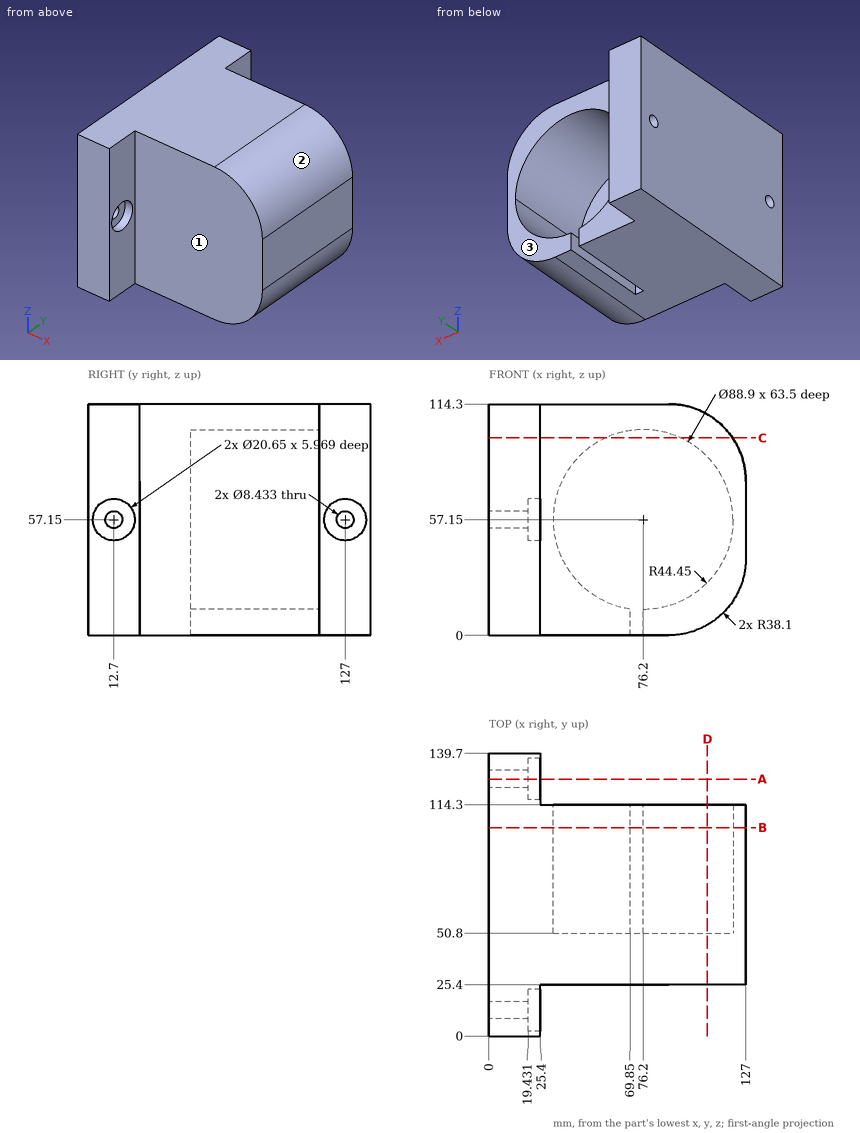
Check sheet for the drawn part. Datum: minimum x, y, z corner. Units: mm. A direction names the side the tool comes from. Give positions to 0.01 mm unless a question says otherwise; leave off trailing zeros. Order: outer loops, then holes, each group sorted by start corner. A loop starts at its lowest first (then second) coordinate and runs counter-clockwise, first axis right, second up. Notation, with made-up numbers: (-33, -18) - (4, -18) arc R15 ccw to (4, -13) - close; hole circle Ø9 at (-13.5, 19). An arc over 180 degrees is marked (long way). Answer in a Markdown table with one row per item. Add a question column.
Q1. Cross-section at B-B, the plane y = 103. Enter the section's corners in (x, z).
Q2. Gauge pin test, flat ends, axial feed: pin 1 (12 mm diameter, centred on y = 16, z = 58.5, fed in from +X); pin 2 (20.5 mm diameter, centred on y = 15, z = 57, fed in from +X); pin 3 (4 mm diameter, centred on x = 85, z = 21, fed in from -Y); pin 4 (4 mm diameter, centred on y = 73, z = 9, fed in from -X). Record the tip position at first contact, or that the pin passes through.
Q3. Tool access check on the marked faces 1, 2 and 3. Record the directions out of +Z, -Z, +X, -X, +Y, -Y that give a thin tool (end or side, any length) a straight path to the whole face; none if there is none.
Q4. Cross-section at D-D, the plane x = 108. Enter the section's corners in (y, z).
Q5. Cross-section at A-A, the plane y = 127. Enter the section's corners in (x, z) (1 decimal).
Q6. Material ranges on probe 1 along Y at (x, z) = (24, 57); probe 2 along X at (y, z) = (101.5, 82.5) (1 decimal); probe 3 along X at (y, z) = (93, 57), recorded low to high. Write a range as from..to.
Q7. Cross-section at C-C, the plane z = 97.5. Enter the section's corners in (x, y).
Check values:
| question | item | result |
|---|---|---|
| 1 | outline | (0, 0) - (69.85, 0) - (69.85, 13.16) arc R44.45 cw (long way) to (76.2, 12.7) - (76.2, 0) - (88.9, 0) arc R38.1 ccw to (127, 38.1) - (127, 76.2) arc R38.1 ccw to (88.9, 114.3) - (0, 114.3) - close |
| 2 | pin 1 | stops at x = 19.43 |
| 2 | pin 2 | stops at x = 25.4 |
| 2 | pin 3 | stops at y = 25.4 |
| 2 | pin 4 | stops at x = 0 |
| 3 | face 1 | +Z, -Z, +X, -Y |
| 3 | face 2 | +Z, +X, +Y, -Y |
| 3 | face 3 | +Z, -Z, +X, +Y |
| 4 | outline | (25.4, 5.13) - (114.3, 5.13) - (114.3, 26.09) - (50.8, 26.09) - (50.8, 88.21) - (114.3, 88.21) - (114.3, 109.17) - (25.4, 109.17) - close |
| 5 | outline | (0, 0) - (25.4, 0) - (25.4, 46.8) - (19.4, 46.8) - (19.4, 52.9) - (0, 52.9) - close; (0, 61.4) - (19.4, 61.4) - (19.4, 67.5) - (25.4, 67.5) - (25.4, 114.3) - (0, 114.3) - close |
| 6 | probe 1 | y = 0..2.38, 23.02..116.68, 137.32..139.7 |
| 6 | probe 2 | x = 0..39.7, 112.7..126.5 |
| 6 | probe 3 | x = 0..31.75, 120.65..127 |
| 7 | outline | (0, 0) - (25.4, 0) - (25.4, 25.4) - (120.49, 25.4) - (120.49, 114.3) - (94.85, 114.3) - (94.85, 50.8) - (57.55, 50.8) - (57.55, 114.3) - (25.4, 114.3) - (25.4, 139.7) - (0, 139.7) - close |
